```python
from build123d import *

# Parameters (mm, degrees)
BOSS_EXTRUDE1_DEPTH = 0.625
CUT_EXTRUDE3_DEPTH  = 0.625
FILLET1_START       = -1
FILLET1_DEPTH       = 3
CUT_EXTRUDE4_REACH  = 81.183
SKETCH5_R           = 1


with BuildPart() as part:
    # Sketch2 → Boss-Extrude1 (new body)
    with BuildSketch(Plane(origin=(0, 0, 0), x_dir=(1, 0, 0), z_dir=(0, 1, 0))):
        with BuildLine():
            Line((8.997858244, -0.196333965), (9.856747342, 39.165996151))
            ThreePointArc((9.856747342, 39.165996151), (9.733712071, 39.668799805), (9.375758573, 40.042722907))
            Line((9.375758573, 40.042722907), (5.794249139, 42.216036183))
            ThreePointArc((5.794249139, 42.216036183), (4.383630471, 43.673589393), (3.869342172, 45.635683666))
            Line((3.869342172, 45.635683666), (3.869342172, 77.038914875))
            ThreePointArc((3.869342172, 77.038914875), (3.676362717, 77.629438236), (3.171906493, 77.992043844))
            ThreePointArc((3.171906493, 77.992043844), (-6.282617519, 76.39229695), (-10.480917414, 67.771305568))
            Line((-10.480917414, 67.771305568), (-8.997858244, -0.196333965))
            ThreePointArc((-8.997858244, -0.196333965), (0, -9), (8.997858244, -0.196333965))
        make_face()
    extrude(amount=BOSS_EXTRUDE1_DEPTH)

    # Sketch3 → Cut-Extrude3 (cut)
    with BuildSketch(Plane(origin=(0, 0.625, 0), x_dir=(1, 0, 0), z_dir=(0, 1, 0))):
        with BuildLine():
            Line((-8.997858244, -0.196333965), (-10.481573544, 67.803666035))
            ThreePointArc((-10.481573544, 67.803666035), (-3.525742077, 56.156825546), (-1.104262014, 42.808832473))
            Line((-1.104262014, 42.808832473), (-1.104262014, 10.808832473))
            ThreePointArc((-1.104262014, 10.808832473), (-3.281700426, 4.037153402), (-8.997858244, -0.196333965))
        make_face()
    extrude(amount=-CUT_EXTRUDE3_DEPTH, mode=Mode.SUBTRACT)


with BuildPart() as body_2:
    # of the pieces the cut leaves, the one that is kept (cut_extrude3_keep)
    add(part.part.solids().sort_by_distance((8.997858244, 0, 0.196333965))[0])

    # Fillet1: read off the stored shape, not the designer's step
    # Fillet1 outline → Fillet1 (cut)
    with BuildSketch(Plane(origin=(0, 0, 0), x_dir=(1, 0, 0), z_dir=(0, 1, 0)).offset(FILLET1_START)):
        with BuildLine():
            ThreePointArc((3.171906493, 77.992043844), (2.204919962, 78.248915013), (1.217849838, 78.412433565))
            ThreePointArc((1.217849838, 78.412433565), (3.110493996, 77.427046766), (3.869342172, 75.432745259))
            Line((3.869342172, 75.432745259), (3.869342172, 77.038914875))
            ThreePointArc((3.869342172, 77.038914875), (3.676362717, 77.629438236), (3.171906493, 77.992043844))
        make_face()
    extrude(amount=FILLET1_DEPTH, mode=Mode.SUBTRACT)

    # Sketch5 → Cut-Extrude4 (cut, up to next)
    with BuildSketch(Plane.XZ, mode=Mode.PRIVATE) as cut_extrude4_sk1:
        with Locations(Location((-5.399070001, -69.616613762, 0), (0, 0, 270))):
            Circle(SKETCH5_R)
    cut_extrude4_tool1 = extrude(cut_extrude4_sk1.sketch, amount=-CUT_EXTRUDE4_REACH, mode=Mode.PRIVATE) & body_2.part
    # Sketch5 → Cut-Extrude4 (cut, up to next)
    with BuildSketch(Plane.XZ, mode=Mode.PRIVATE) as cut_extrude4_sk2:
        with Locations(Location((6.76984482, -35.216036183, 0), (0, 0, 270))):
            Circle(SKETCH5_R)
    cut_extrude4_tool2 = extrude(cut_extrude4_sk2.sketch, amount=-CUT_EXTRUDE4_REACH, mode=Mode.PRIVATE) & body_2.part
    # Sketch5 → Cut-Extrude4 (cut, up to next)
    with BuildSketch(Plane.XZ, mode=Mode.PRIVATE) as cut_extrude4_sk3:
        with Locations(Location((-2.705062156, -1.67, 0), (0, 0, 270))):
            Circle(SKETCH5_R)
    cut_extrude4_tool3 = extrude(cut_extrude4_sk3.sketch, amount=-CUT_EXTRUDE4_REACH, mode=Mode.PRIVATE) & body_2.part
    add(cut_extrude4_tool1.solids().sort_by_distance((-5.39907, 0, -69.616614))[0], mode=Mode.SUBTRACT)
    add(cut_extrude4_tool2.solids().sort_by_distance((6.769845, 0, -35.216036))[0], mode=Mode.SUBTRACT)
    add(cut_extrude4_tool3.solids().sort_by_distance((-2.705062, 0, -1.67))[0], mode=Mode.SUBTRACT)


solid = body_2.part
```
Could you check a few things on this model? Use its own coordinates, in mm. A direction names the side the tool comes from. Give positions to 0.01 mm unless a question says otherwise; leave off trailing zeros. Write each loop counter-clockwise with the first axis right and the second up, starting at its lowest first coordinate (ties: lowest second). Pieces come first, ordered by that corner, then holes. Notation, with made-up numbers: (82, 20.5) -> (105, 20.5) arc R30 ccw to (105, 42.5) -> close; hole circle Ø6 at (32, -0.5). An arc over 180 degrees is marked (long way). Write each question's results on one line, items separated by ' | '.
1. If we mould it in two halves opening along X, with no side actions, what happens to faces 1 (the cylindrical face through (-0.195, 0.308, 8.998)), 2 (the cylindrical face through (-3.593, 0.317, -56.335)), 3 (the cylindrical face through (4.398, 0.308, -43.649)), 4 (the cylindrical face through (6.814, 0.308, -34.217))? For each: released by +X, released by -X, zero draft, split by the parting line, or undercut.
Check sheet entries:
face 1: split by the parting line | face 2: released by -X | face 3: released by +X | face 4: undercut
2. I want a section at B-B, the plane y = 0.2. Write out the boundary of the cut face in (x, z), then the cut area to 3 significant figures.
Check sheet entries:
outline: (-10.48, -67.8) arc R10.48 ccw to (1.22, -78.41) arc R3 ccw to (3.87, -75.43) -> (3.87, -45.64) arc R4 cw to (5.79, -42.22) -> (9.38, -40.04) arc R1 ccw to (9.86, -39.17) -> (9, 0.2) arc R9 ccw to (-9, 0.2) arc R11.62 cw to (-1.1, -10.81) -> (-1.1, -42.81) arc R38 cw to start; hole circle Ø2 at (-5.4, -69.62); hole circle Ø2 at (-2.71, -1.67); hole circle Ø2 at (6.77, -35.22) | area: 911 mm²
3. I need wall thicknesses on L1, parallel to Z at x = -5.5, y = 0.55; L2, parallel to Z at x = -6.75, y = 0.55; L3, parallel to X at y = 0.5, z = -1.67. Which ranges of each line are inside material? Lowest first, please.
Check sheet entries:
L1: z = -76.92 to -70.61, -68.62 to -60.55, -1.71 to 7.12 | L2: z = -76.02 to -62.74, -0.84 to 5.95 | L3: x = -5.55 to -3.71, -1.71 to 9.04
4. Will this pin go through, and if not, where does the flat tip stop? pin 1 Ø1.2 at (x, z) = (-5.4, -69.62) entering from -Y.
Check sheet entries:
pin 1: passes through
5. I want a section at A-A, the plane z = -1.67. Write out the boundary of the cut face in (x, y) (3 decimals), then the cut area to 3 significant figures.
Check sheet entries:
outline: (-5.548, 0) -> (-3.705, 0) -> (-3.705, 0.625) -> (-5.548, 0.625) -> close; (-1.705, 0) -> (9.039, 0) -> (9.039, 0.625) -> (-1.705, 0.625) -> close | area: 7.87 mm²
6. I want a section at C-C, the plane z = -28. Write out the boundary of the cut face in (x, y) (3 decimals), then the cut area to 3 significant figures.
Check sheet entries:
outline: (-1.104, 0) -> (9.613, 0) -> (9.613, 0.625) -> (-1.104, 0.625) -> close | area: 6.70 mm²
7. On a 3-axis mill with a long thin cutter (end or side, diameter ignored), from which of +Z, -Z, +X, -X, +Y, -Y can I reach the whole of each face in a straight line? I mean faces 5 (the cylindrical face through (-2.405, 0.308, -2.624)), 6 (the cylindrical face through (-3.223, 0.317, -4.12)). Say none if no direction works.
Check sheet entries:
face 5: +Y, -Y | face 6: -X, +Y, -Y
8. I want a section at D-D, the plane z = -53. Write out the boundary of the cut face in (x, y) (3 decimals), then the cut area to 3 significant figures.
Check sheet entries:
outline: (-2.496, 0) -> (3.869, 0) -> (3.869, 0.625) -> (-2.496, 0.625) -> close | area: 3.98 mm²
